Can you work these out from the drawing? Everything is in mm from the part's minimum corner. A direction names the side the tool comes from. Give positions to 0.01 mm unless a question says otherwise; leave off trailing zeros. Order: outer loops, then holes, each group sorted by start corner. A loop starts at its lowest first (then second) coordinate and runs counter-clockwise, first axis right, second up. Notation, with made-up numbers: M 89.5,-16 L 117.5,-16 A11 cw 117.5,1 Z; hole C 55,36.25 d2. An arc over 180 degrees is marked long. Use a Markdown table: item, result. Add a question column.
Item 1: I'm going to push flat-ended pins straight in: pin 1 Ø6 at (x, z) = (10.5, 34) entering from +Y; pin 2 Ø2.5 at (y, z) = (10, 31) entering from -X; pin 3 Ø2.5 at (y, z) = (7.5, 18) entering from +X. Where does each tip first touch, or does it pass through?
Item 2: If I drill on L1, parallel to Z at x = 1.25, y = 10; L2, parallel to X at y = 14.5, z = 12.5; L3, parallel to Y at x = 19, z = 4, over which ranges is the centre line in solid material (lowest first)? Write a range as from..to.
Item 3: For the marked faces 5 and 6, which set-ups out of +Z, -Z, +X, -X, +Y, -Y let a thin tool reach every point of the face, with its end or its side?
Item 4: Suppose I cut it at D-D on z = 37. Write out the boundary of the cut face in (x, y), plus the area to 3 significant figures.
Item 5: Suppose I cut it at C-C on y = 5.5. Write out the boundary of the cut face in (x, z).
Item 6: Suppose I cut it at A-A on y = 7.5. Write out the boundary of the cut face in (x, z).
Item 7: If we mould it in two halves opening along X, with no side actions, what happens to the marked faces 1, 2, 3 and 4? For each: released by +X, released by -X, zero draft, split by the parting line, or undercut.
Item 8: Suppose I cut it at B-B on z = 4. Write out the boundary of the cut face in (x, y).
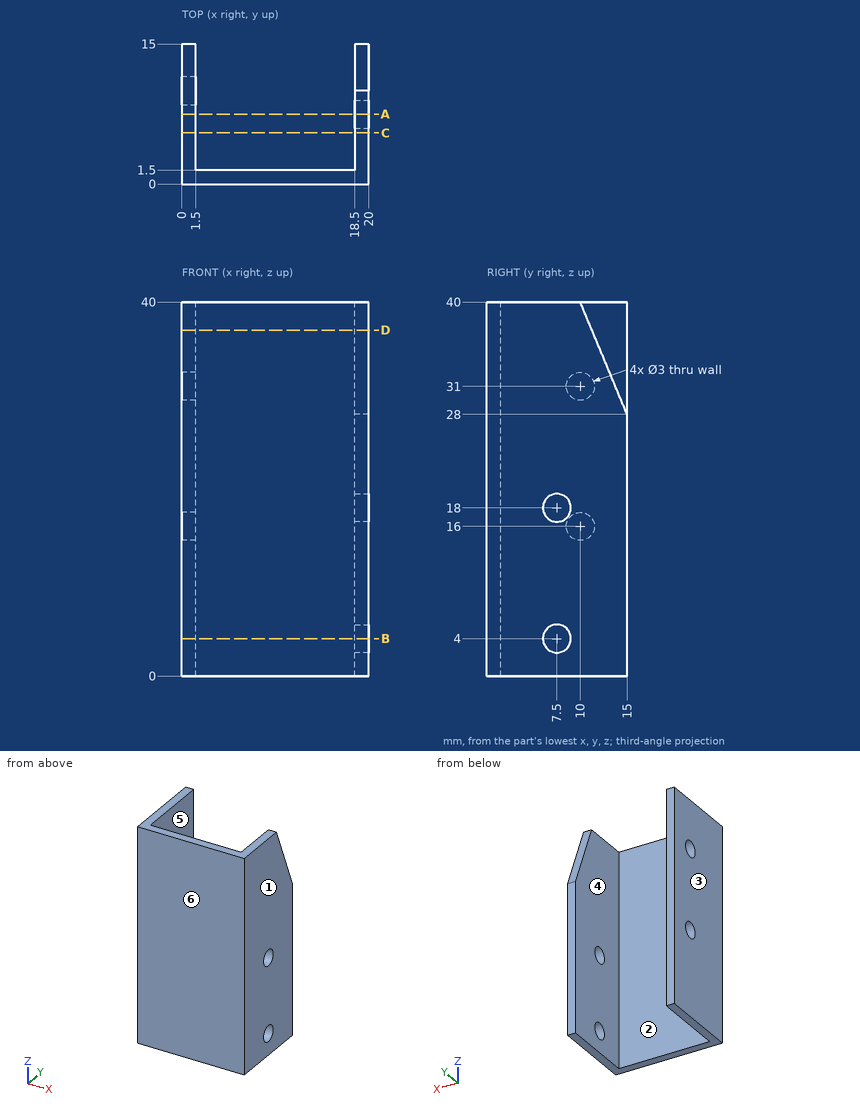
Findings below:
| question | item | result |
|---|---|---|
| 1 | pin 1 | stops at y = 1.5 |
| 1 | pin 2 | stops at x = 18.5 |
| 1 | pin 3 | stops at x = 1.5 |
| 2 | L1 | z = 0..14.5, 17.5..29.5, 32.5..40 |
| 2 | L2 | x = 0..1.5, 18.5..20 |
| 2 | L3 | y = 0..6, 9..15 |
| 3 | face 5 | +Z, -Z, +Y |
| 3 | face 6 | +Z, -Z, +X, -X, -Y |
| 4 | outline | M 0,0 L 20,0 L 20,11.25 L 18.5,11.25 L 18.5,1.5 L 1.5,1.5 L 1.5,15 L 0,15 Z |
| 4 | area | 64.9 mm^2 |
| 5 | outline | M 0,0 L 1.5,0 L 1.5,40 L 0,40 Z; M 18.5,0 L 20,0 L 20,40 L 18.5,40 Z |
| 6 | outline | M 0,0 L 1.5,0 L 1.5,40 L 0,40 Z; M 18.5,0 L 20,0 L 20,2.5 L 18.5,2.5 Z; M 18.5,5.5 L 20,5.5 L 20,16.5 L 18.5,16.5 Z; M 18.5,19.5 L 20,19.5 L 20,40 L 18.5,40 Z |
| 7 | face 1 | released by +X |
| 7 | face 2 | undercut |
| 7 | face 3 | released by -X |
| 7 | face 4 | undercut |
| 8 | outline | M 0,0 L 20,0 L 20,6 L 18.5,6 L 18.5,1.5 L 1.5,1.5 L 1.5,15 L 0,15 Z; M 18.5,9 L 20,9 L 20,15 L 18.5,15 Z |
